Can you work these out from the model? Positions are in its coordinate system, mm. A direction names the side the tool comes from. Coordinates: 2 decimals unless noted, no trailing zeros. Write each loop counter-clockwise with the first axis right and the second up, starting at its lowest first coordinate (ties: lowest second). Pieces come first, ordered by that corner, then holes. Notation, with made-up numbers: (9.5, 73) - (32.5, 73) arc R16 ccw to (32.5, 104) - close; hole circle Ø5 at (-4, 15). An arc over 180 degrees is marked (long way). One line per question, with ' | ' between items. Start each with the question number.
from build123d import *

# Parameters (mm, degrees)
F1_DEPTH = 25.4


with BuildPart() as f1:
    # F0 (on Front) → F1 (new body)
    with BuildSketch(Plane.XZ):
        Polygon((17.3676, 4.654796), (10.548249, 42.882821), (4.823116, 6.63619), align=None)
        Polygon((-20.812961, -22.530177), (4.823116, 6.63619), (-27.085203, -11.487125), align=None)
        Polygon((-65.872219, -9.628965), (-27.085203, -11.487125), (-61.149093, 2.160101), align=None)
        Polygon((-83.879634, 33.643555), (-61.149093, 2.160101), (-71.71775, 37.301229), align=None)
        Polygon((-71.71775, 37.301229), (-50.832759, 67.474272), (-61.275255, 74.702294), align=None)
        Polygon((-50.832759, 67.474272), (-14.220945, 69.958314), (-15.08064, 82.629184), align=None)
        Polygon((-14.220945, 69.958314), (10.548249, 42.882821), (19.918723, 51.455114), align=None)
        Polygon((4.823116, 6.63619), (10.548249, 42.882821), (-14.220945, 69.958314), (-50.832759, 67.474272), (-71.71775, 37.301229), (-61.149093, 2.160101), (-27.085203, -11.487125), align=None)
    extrude(amount=F1_DEPTH)


solid = f1.part
(1) If we section it at A-A on y = -21.5: List the corners of the cut face in (x, z) for me, plus the area to 3 significant figures.
(2) If we section it at B-B on x = 1: List the corners of the cut face in (y, z) for me, plus the area to 3 significant figures.
(3) If we section it at C-C on z = 53.5: List the corners of the cut face in (x, y) for me (3 decimals).
(4) If we mould it in two halves opening along Z, with no side actions, what happens to faces 6 (the face through (-55.981, -12.522, 71.038)), 7 (the face through (-23.993, -12.522, -16.931)), 8 (the face through (-72.67, -12.52, 18.12)), 9 (the face through (-63.478, -12.522, -3.652))? For each: +Z half, -Z half, draft (parallel to the pull), parting line (faces both ways), or undercut.
(5) Which directions (+Z, -Z, +X, -X, +Y, -Y) give clear straight access to the entire face, cutting with the end or side of a thin tool? Please do faces 1 (the face through (-33, -25.4, 31)), 2 (the face through (-46.75, -12.522, -10.545)), 3 (the face through (14.006, -12.522, 23.501)), 4 (the face through (-32.706, -12.522, 75.158)), 5 (the face through (11.01, -12.52, 5.66)).
(6) I'm going to push flat-ended pins straight in: pin 1 (10 mm diameter, centred on x = -13.5, y = -16.5, fed in from -Z); pin 2 (5 mm diameter, centred on y = -4.5, z = 14, fed in from -X); pin 3 (8 mm diameter, centred on y = -12, z = -5.5, fed in from -X). Where does each tip first touch, or does it pass through?
(7) If I drill on probe 1 along X at (y, z) = (-9, 71); probe 2 along X at (y, z) = (-5.75, 71.5); probe 3 along Z at (x, y) = (-17.5, -7.75), over which ranges is the centre line in solid material (lowest first)?
Values:
1) outline: (-83.88, 33.64) - (-61.15, 2.16) - (-65.87, -9.63) - (-27.09, -11.49) - (-20.81, -22.53) - (4.82, 6.64) - (17.37, 4.65) - (10.55, 42.88) - (19.92, 51.46) - (-14.22, 69.96) - (-15.08, 82.63) - (-50.83, 67.47) - (-61.28, 74.7) - (-71.72, 37.3) - close | area: 6,520 mm2
2) outline: (-25.4, 2.29) - (0, 2.29) - (0, 61.71) - (-25.4, 61.71) - close | area: 1,510 mm2
3) outline: (-67.195, -25.4) - (16.146, -25.4) - (16.146, 0) - (-67.195, 0) - close
4) face 6: +Z half | face 7: -Z half | face 8: undercut | face 9: undercut
5) face 1: +Z, -Z, +X, -X, -Y | face 2: -Z, -X, +Y, -Y | face 3: +X, +Y, -Y | face 4: +Z, +Y, -Y | face 5: -Z, +Y, -Y
6) pin 1: z = -19.9 | pin 2: x = -71.5 | pin 3: x = -65.82
7) probe 1: -62.31 to -55.93, -42.52 to -14.29 | probe 2: -62.17 to -56.65, -41.34 to -14.33 | probe 3: -18.76 to 81.6
